Can you work these out from the model? Positions are in its coordinate system, mm. Coordinates: 2 decimals unless noted, no trailing zeros. Loops run counter-clockwise (first coordinate to the right, second up) from the corner with the lowest first, then second, coordinate; pieces in that order, holes last. Notation, with made-up numbers: (50, 78) -> (91, 78) arc R20 cw to (91, 109) -> close; hole circle Ø5 at (20.5, -36.5). An arc over 180 degrees is marked (long way). Use one line per item in the form item = value. Start each with the question number.
(1) Imagine slicing it at B-B (x = -30). List the corners of the cut face in (y, z) for me, plus the area to 3 significant figures.
(2) Imagine slicing it at A-A (y = -12). List the corners of the cut face in (x, z) for me (3 decimals).
(3) I'm going to push flat-ended pins straight in: pin 1 (5 mm diameter, centred on x = 12.5, z = 1, fed in from +Y); pin 2 (4 mm diameter, centred on x = 16, z = 3.5, fed in from +Y); pin 3 (1 mm diameter, centred on x = 11.5, y = -1, fed in from -Z); pin 4 (1 mm diameter, centred on x = 10.5, z = -3.5, fed in from +Y). Where does each tip first touch, or does it pass through?
(4) I need wall thicknesses on line 1 (Y direction, x = -30, z = 2.5); line 2 (X direction, y = 9, z = -3.5); line 3 (X direction, y = -15.5, z = -0.25). Which ranges of each line are inside material? Lowest first, please. Write a range as [from, to].
(5) Thinking about a two-plate mould opening in Y: for faces 1 (the cylindrical face through (-21.47, 19.9, 0.07)), 2 (the cylindrical face through (24.052, 16.045, 0.07)), 3 (the flat face through (0, -8, 0)), which applies, released by +Y, released by -Y, zero draft, split by the parting line, or undercut?
(6) Imagine slicing it at C-C (y = 10). List the corners of the cut face in (x, z) for me, plus the area to 3 significant figures.
(7) Imagine slicing it at D-D (z = -3). List the corners of the cut face in (x, y) for me (3 decimals).
```python
from build123d import *

# Parameters (mm, degrees)
EXTRUDE_1_DEPTH          = 5
FILLET_1_R               = 2
FILLET_2_R               = 2
SKETCH_2_R               = 2.025
CUT_EXTRUDE_1_DEPTH      = 11
SKETCH_3_W               = 25
SKETCH_3_H               = 6
CUT_EXTRUDE_2_DEPTH      = 11
FILLET_3_R               = 2
SKETCH_4_R               = 2.15
CUT_EXTRUDE_3_DEPTH      = 1
CUT_EXTRUDE_3_DEPTH_BACK = 11
SKETCH_5_R               = 2.15
CUT_EXTRUDE_4_DEPTH      = 1
CUT_EXTRUDE_4_DEPTH_BACK = 11


with BuildPart() as part:
    # 草图1 → 凸台-拉伸1 (new body, symmetric)
    with BuildSketch(Plane.XY):
        with BuildLine():
            Line((0, 0), (0, -24))
            Line((0, -24), (25, -24))
            Line((25, -24), (25, 17.926801262))
            ThreePointArc((25, 17.926801262), (3.142873043, 13.301970467), (-15.238723859, 26))
            Line((-15.238723859, 26), (-35, 26))
            Line((-35, 26), (-35, 6))
            Line((-35, 6), (-7, 6))
            Line((-7, 6), (0, 0))
        make_face()
    extrude(amount=EXTRUDE_1_DEPTH, both=True)

    # 圆角1
    fillet_1_edges = [part.edges().sort_by_distance(p)[0] for p in [
        (-7, 6, 0),
        (-35, 6, 0),
        (-35, 26, 0),
        (25, -24, 0),
        (0, -24, 0),
        (0, 0, 0),
    ]]
    fillet(fillet_1_edges, radius=FILLET_1_R)

    # 圆角2
    fillet_2_edges = [part.edges().sort_by_distance(p)[0] for p in [
        (-15.238723859, 26, 0),
        (25, 17.926801262, 0),
    ]]
    fillet(fillet_2_edges, radius=FILLET_2_R)

    # 草图2 → 切除-拉伸1 (cut, through all)
    with BuildSketch(Plane.XY.offset(5)):
        with Locations((12.5, -2)):
            Circle(SKETCH_2_R)
        with Locations((12.5, -12)):
            Circle(SKETCH_2_R)
    extrude(amount=-CUT_EXTRUDE_1_DEPTH, mode=Mode.SUBTRACT)

    # 草图3 → 切除-拉伸2 (cut, through all)
    with BuildSketch(Plane.XY.offset(5)):
        with Locations((12.5, -21)):
            Rectangle(SKETCH_3_W, SKETCH_3_H)
    extrude(amount=-CUT_EXTRUDE_2_DEPTH, mode=Mode.SUBTRACT)

    # 圆角3
    fillet_3_edges = [part.edges().sort_by_distance(p)[0] for p in [
        (0, -18, 0),
        (25, -18, 0),
    ]]
    fillet(fillet_3_edges, radius=FILLET_3_R)

    # 草图4 → 切除-拉伸3 (cut, two sides)
    with BuildSketch(Plane.XY.offset(5)) as cut_extrude_3_sk:
        with Locations((-30, 22)):
            Circle(SKETCH_4_R)
        with Locations((-30, 10)):
            Circle(SKETCH_4_R)
    extrude(amount=CUT_EXTRUDE_3_DEPTH, mode=Mode.SUBTRACT)
    extrude(cut_extrude_3_sk.sketch, amount=-CUT_EXTRUDE_3_DEPTH_BACK, mode=Mode.SUBTRACT)

    # 草图5 → 切除-拉伸4 (cut, two sides)
    with BuildSketch(Plane.XY.offset(5)) as cut_extrude_4_sk:
        with Locations((-21, 10)):
            Circle(SKETCH_5_R)
        with Locations((-21, 22)):
            Circle(SKETCH_5_R)
    extrude(amount=CUT_EXTRUDE_4_DEPTH, mode=Mode.SUBTRACT)
    extrude(cut_extrude_4_sk.sketch, amount=-CUT_EXTRUDE_4_DEPTH_BACK, mode=Mode.SUBTRACT)


solid = part.part
```
Worked out:
q1.outline = (6, -5) -> (7.85, -5) -> (7.85, 5) -> (6, 5) -> close; (12.15, -5) -> (19.85, -5) -> (19.85, 5) -> (12.15, 5) -> close; (24.15, -5) -> (26, -5) -> (26, 5) -> (24.15, 5) -> close
q1.area = 114 mm2
q2.outline = (0, -5) -> (10.475, -5) -> (10.475, 5) -> (0, 5) -> close; (14.525, -5) -> (25, -5) -> (25, 5) -> (14.525, 5) -> close
q3.pin_1 = 13.46
q3.pin_2 = 14.32
q3.pin_3 = through
q3.pin_4 = 12.84
q4.line_1 = [6, 7.85], [12.15, 19.85], [24.15, 26]
q4.line_2 = [-35, -31.9], [-28.1, -22.9], [-19.1, 25]
q4.line_3 = [0, 25]
q5.face_1 = undercut
q5.face_2 = released by +Y
q5.face_3 = zero draft
q6.outline = (-35, -5) -> (-32.15, -5) -> (-32.15, 5) -> (-35, 5) -> close; (-27.85, -5) -> (-23.15, -5) -> (-23.15, 5) -> (-27.85, 5) -> close; (-18.85, -5) -> (25, -5) -> (25, 5) -> (-18.85, 5) -> close
q6.area = 514 mm2
q7.outline = (-35, 8) arc R2 ccw to (-33, 6) -> (-7.74, 6) arc R2 cw to (-6.438, 5.519) -> (-0.698, 0.599) arc R2 cw to (0, -0.92) -> (0, -16) arc R2 ccw to (2, -18) -> (23, -18) arc R2 ccw to (25, -16) -> (25, 14.343) arc R2 ccw to (22.055, 16.106) arc R28.25 cw to (-14.667, 25.124) arc R2 ccw to (-16.321, 26) -> (-33, 26) arc R2 ccw to (-35, 24) -> close; hole circle Ø4.3 at (-30, 10); hole circle Ø4.3 at (-30, 22); hole circle Ø4.3 at (-21, 10); hole circle Ø4.3 at (-21, 22); hole circle Ø4.05 at (12.5, -12); hole circle Ø4.05 at (12.5, -2)
